from build123d import *

# Parameters (mm, degrees)
SKETCH1_W           = 82.042
SKETCH1_H           = 50.8
BOSS_EXTRUDE1_DEPTH = 31.242
SKETCH2_W           = 66.04
SKETCH2_H           = 45.72
CUT_EXTRUDE1_DEPTH  = 30.48
SKETCH3_R           = 3
CUT_EXTRUDE2_DEPTH  = 58.479953071
SKETCH4_W           = 8.001
SKETCH4_H           = 15.711289628
CUT_EXTRUDE3_DEPTH  = 30.48
SKETCH5_R           = 3
CUT_EXTRUDE4_DEPTH  = 58.069368675
SKETCH6_W           = 30.008710372
SKETCH6_H           = 24.13
CUT_EXTRUDE5_DEPTH  = 92.389891826
BOSS_EXTRUDE2_DEPTH = 2.54
BOSS_EXTRUDE3_DEPTH = 2.54


with BuildPart() as part:
    # Sketch1 → Boss-Extrude1 (new body)
    with BuildSketch(Plane(origin=(0, 0, 0), x_dir=(1, 0, 0), z_dir=(0, 1, 0))):
        Rectangle(SKETCH1_W, SKETCH1_H)
    extrude(amount=BOSS_EXTRUDE1_DEPTH)

    # Sketch2 → Cut-Extrude1 (cut)
    with BuildSketch(Plane(origin=(0, 31.242, 0), x_dir=(1, 0, 0), z_dir=(0, 1, 0))):
        with Locations((0, -2.54)):
            Rectangle(SKETCH2_W, SKETCH2_H)
    extrude(amount=-CUT_EXTRUDE1_DEPTH, mode=Mode.SUBTRACT)

    # Sketch3 → Cut-Extrude2 (cut, through all)
    with BuildSketch(Plane(origin=(0, 31.242, 0), x_dir=(1, 0, 0), z_dir=(0, 1, 0))):
        with Locations(Location((-37.5, 13.82, 0), (0, 0, 270))):
            Circle(SKETCH3_R)
        with Locations(Location((-37.5, -3.18, 0), (0, 0, 270))):
            Circle(SKETCH3_R)
        with Locations(Location((37.5, 13.82, 0), (0, 0, 270))):
            Circle(SKETCH3_R)
        with Locations(Location((37.5, -3.18, 0), (0, 0, 270))):
            Circle(SKETCH3_R)
    extrude(amount=-CUT_EXTRUDE2_DEPTH, mode=Mode.SUBTRACT)

    # Sketch4 → Cut-Extrude3 (cut)
    with BuildSketch(Plane(origin=(0, 31.242, 0), x_dir=(1, 0, 0), z_dir=(0, 1, 0))):
        with Locations((-37.0205, -17.544355186)):
            Rectangle(SKETCH4_W, SKETCH4_H)
        with Locations((37.0205, -17.544355186)):
            Rectangle(SKETCH4_W, SKETCH4_H)
    extrude(amount=-CUT_EXTRUDE3_DEPTH, mode=Mode.SUBTRACT)

    # Sketch5 → Cut-Extrude4 (cut, through all)
    with BuildSketch(Plane(origin=(0, 0.762, 0), x_dir=(1, 0, 0), z_dir=(0, 1, 0))):
        with Locations(Location((0, -17.308710372, 0), (0, 0, 270))):
            Circle(SKETCH5_R)
        with Locations(Location((-20.32, -17.308710372, 0), (0, 0, 270))):
            Circle(SKETCH5_R)
        with Locations(Location((20.32, -17.308710372, 0), (0, 0, 270))):
            Circle(SKETCH5_R)
    extrude(amount=-CUT_EXTRUDE4_DEPTH, mode=Mode.SUBTRACT)

    # Sketch6 → Cut-Extrude5 (cut, through all)
    with BuildSketch(Plane(origin=(41.021, 0, 0), x_dir=(0, 0, -1), z_dir=(1, 0, 0))):
        with Locations((5.315644814, 12.827)):
            Rectangle(SKETCH6_W, SKETCH6_H)
    extrude(amount=-CUT_EXTRUDE5_DEPTH, mode=Mode.SUBTRACT)

    # Sketch8 → Boss-Extrude2 (add)
    with BuildSketch(Plane.ZY.offset(41.021)):
        Polygon((9.688710372, 24.892), (9.688710372, 31.242), (-25.4, 31.242), (-25.4, 0), (25.4, 0), (25.4, 0.762), (-20.32, 0.762), (-20.32, 24.892), align=None)
    extrude(amount=BOSS_EXTRUDE2_DEPTH)

    # Sketch9 → Boss-Extrude3 (add)
    with BuildSketch(Plane(origin=(41.021, 0, 0), x_dir=(0, 0, -1), z_dir=(1, 0, 0))):
        Polygon((-9.688710372, 31.242), (-9.688710372, 24.892), (20.32, 24.892), (20.32, 0.762), (-25.4, 0.762), (-25.4, 0), (25.4, 0), (25.4, 31.242), align=None)
    extrude(amount=BOSS_EXTRUDE3_DEPTH)


solid = part.part
Geometry check sheet. Reference: the model listing, model coordinates, mm. A direction names the side the tool comes from. Give positions to 0.01 mm unless a question says otherwise; leave off trailing zeros. Write each loop counter-clockwise with the first axis right and the second up, starting at its lowest first coordinate (ties: lowest second). Pieces come first, ordered by that corner, then holes. Notation, with made-up numbers: M 18.5,49 L 36.5,49 A20 cw 36.5,72 Z; hole C 76,39 d6. An arc over 180 degrees is marked long. One line per question, with ' | ' between items.
1. Scan lines: line 1 along X through (y, z) = (30.25, -13.82); line 2 along X through (y, z) = (0.2, -13.82); line 3 along Z through (x, y) = (-37, 26). Record each from-to range of solid material in increasing order. Write a range as from..to.
Ans:
line 1: -43.56..-40.5, -34.5..-33.02, 33.02..34.5, 40.5..43.56 | line 2: -43.56..-40.5, -34.5..34.5, 40.5..43.56 | line 3: -25.4..-16.78, -10.86..0.22, 6.14..9.69
2. Cross-section at A-A (x = -20.32). Enter the section's corners in (y, z), plus the area to 3 significant figures.
Ans:
outline: M 0,-25.4 L 31.24,-25.4 L 31.24,-20.32 L 0.76,-20.32 L 0.76,14.31 L 0,14.31 Z; M 0,20.31 L 0.76,20.31 L 0.76,25.4 L 0,25.4 Z | area: 189 mm2
3. Set-up check for faces 1 (the face through (-38, 28, 9.689)), 2 (the face through (33.02, 28, -5)), 3 (the face through (-34.97, 0.39, 4.79)), 4 (the face through (-1, 16, -20.32)), 5 (the face through (-3, 31.242, -21)): record each of +Z, -Z, +X, -X, +Y, -Y from which the full face is reachable in a straight line by a thin tool's end or side.
Ans:
face 1: +Z, +X, -X, +Y | face 2: +Z, +Y | face 3: +Y, -Y | face 4: +Z | face 5: +Z, -Z, +X, -X, +Y
4. Mould release check, pull along X, two halves, no side actions. Record for faces 6 (the face through (43.561, 26, -11)), 7 (the face through (-34.97, 28.11, -12.21)), 8 (the face through (38, 28, 9.689)): released by +X, released by -X, zero draft, split by the parting line, or undercut.
Ans:
face 6: released by +X | face 7: undercut | face 8: zero draft
5. Gauge pin test, flat ends, axial feed: pin 1 (5 mm diameter, centred on x = -37.5, z = -13.82, fed in from -Y); pin 2 (5 mm diameter, centred on x = -37, y = 27.5, fed in from +Z); pin 3 (5 mm diameter, centred on x = 30.5, y = 20, fed in from +Z); pin 4 (13.5 mm diameter, centred on x = -0.5, z = 6.5, fed in from +Y). Record the tip position at first contact, or that the pin passes through.
Ans:
pin 1: through | pin 2: z = 9.69 | pin 3: z = -20.32 | pin 4: y = 0.76
6. Cross-section at C-C (y = 28). Enter the section's corners in (x, z), plus the area to 3 significant figures.
Ans:
outline: M -43.56,-25.4 L 43.56,-25.4 L 43.56,9.69 L 33.02,9.69 L 33.02,-20.32 L -33.02,-20.32 L -33.02,9.69 L -43.56,9.69 Z; hole C -37.5,-13.82 d6; hole C -37.5,3.18 d6; hole C 37.5,-13.82 d6; hole C 37.5,3.18 d6 | area: 962 mm2
7. Cross-section at D-D (x = 37.5). Enter the section's corners in (y, z), plus the area to 3 significant figures.
Ans:
outline: M 0,-25.4 L 31.24,-25.4 L 31.24,-16.82 L 24.89,-16.82 L 24.89,-20.32 L 0.76,-20.32 L 0.76,-16.82 L 0,-16.82 Z; M 0,-10.82 L 0.76,-10.82 L 0.76,0.18 L 0,0.18 Z; M 0,6.18 L 0.76,6.18 L 0.76,25.4 L 0,25.4 Z; M 24.89,-10.82 L 31.24,-10.82 L 31.24,0.18 L 24.89,0.18 Z; M 24.89,6.18 L 31.24,6.18 L 31.24,9.69 L 24.89,9.69 Z | area: 299 mm2
8. Cross-section at B-B (z = 8). Enter the section's corners in (x, y).
Ans:
outline: M -43.56,0 L 43.56,0 L 43.56,0.76 L -43.56,0.76 Z; M -43.56,24.89 L -33.02,24.89 L -33.02,31.24 L -43.56,31.24 Z; M 33.02,24.89 L 43.56,24.89 L 43.56,31.24 L 33.02,31.24 Z
